Check sheet for the modelled part. Datum: model origin and axes. Units: mm. A direction names the side the tool comes from. Round coordinates to 2 decimals unless told otherwise and drop trailing zeros. Loops run counter-clockwise (first coordinate to the right, second up) from the corner with the lowest first, then second, coordinate; pieces in that order, holes last. Notation, with made-up numbers: (-36, -28.75) - (10, -28.75) arc R27 cw to (10, 8.25) - close; hole circle Ø1 at (-34, 14.25). An arc over 180 degrees is marked (long way). Put each result on its own line as item: value. Start each with the question number.
Item 1: Section check A-A, the plane x = 21. Record the cut outline in (y, z).
Item 2: Section check C-C, the plane z = 23. Record the cut outline in (x, y), and give its area (3 significant figures).
Item 3: Section check D-D, the plane y = 36.5. Record the cut outline in (x, z).
Item 4: Tool access check on faces 4 (the flat face through (21, -19.2, 24)), 5 (the cylindrical face through (37.34, -21.19, 20.89)), 6 (the flat face through (21, -11, 40)). Record the directions out of +Z, -Z, +X, -X, +Y, -Y that give a thin tool (end or side, any length) a straight path to the whole face; none if there is none.
Item 5: Draft check along Y on faces 1 (the cylindrical face through (37.215, 35.125, 1.479)), 2 (the flat face through (16, 19, 3)), 3 (the flat face through (21, -19.2, 45)). Enter one of: pulls with the +Y half, pulls with the -Y half, needs draft (parallel to the pull), parting line crosses it, or undercut.
Item 6: Material ranges on line 1 along X through (y, z) = (-21.25, 23); line 2 along Y through (x, z) = (36.5, 2.1); line 3 along Z through (x, y) = (36, -21), recorded low to high.
Item 7: Section check B-B, the plane y = -16. Record the cut outline in (x, z), and give its area (3 significant figures).
Item 8: Gauge pin test, flat ends, axial feed: pin 1 Ø2 at (x, z) = (28, 22.5) entering from +Y; pin 2 Ø13.5 at (x, y) = (12.5, -6.5) entering from +Z; pin 3 Ø12 at (x, y) = (26, 6.5) entering from +Z. Record the tip position at first contact, or that the pin passes through.
from build123d import *

# Parameters (mm, degrees)
ESQUISSE1_W             = 42
ESQUISSE1_H             = 42
ESQUISSE1_R             = 2.6
ESQUISSE1_R_2           = 1.55
ESQUISSE1_H_2           = 22.2
BOSS_EXTRU_1_DEPTH      = 3
ESQUISSE2_W             = 42
ESQUISSE2_H             = 3
BOSS_EXTRU_2_DEPTH      = 48
BOSS_EXTRU_3_DEPTH      = 42
ENL_V_MAT_EXTRU_4_REACH = 5
ESQUISSE4_R             = 2.5
CHANFREIN1_SIZE         = 1
ESQUISSE5_W             = 42
ESQUISSE5_H             = 10
BOSS_EXTRU_4_DEPTH      = 17


with BuildPart() as part:
    # Esquisse1 → Boss.-Extru.1 (new body)
    with BuildSketch(Plane.XY):
        with Locations((21, 21)):
            Rectangle(ESQUISSE1_W, ESQUISSE1_H)
        with Locations((21, 21)):
            Circle(ESQUISSE1_R, mode=Mode.SUBTRACT)
        with Locations((5.5, 36.5)):
            Circle(ESQUISSE1_R_2, mode=Mode.SUBTRACT)
        with Locations((36.5, 36.5)):
            Circle(ESQUISSE1_R_2, mode=Mode.SUBTRACT)
        with Locations((36.5, 5.5)):
            Circle(ESQUISSE1_R_2, mode=Mode.SUBTRACT)
        with Locations((5.5, 5.5)):
            Circle(ESQUISSE1_R_2, mode=Mode.SUBTRACT)
        with Locations((21, -11.1)):
            Rectangle(ESQUISSE1_W, ESQUISSE1_H_2)
    extrude(amount=BOSS_EXTRU_1_DEPTH)

    # Esquisse2 → Boss.-Extru.2 (add)
    with BuildSketch(Plane.XY.offset(3)):
        with Locations((21, -20.7)):
            Rectangle(ESQUISSE2_W, ESQUISSE2_H)
    extrude(amount=BOSS_EXTRU_2_DEPTH)

    # Esquisse3 → Boss.-Extru.3 (add)
    with BuildSketch(Plane(origin=(42, 0, 0), x_dir=(0, 0, -1), z_dir=(1, 0, 0))):
        Polygon((-3, -4.2), (-18, -19.2), (-3, -19.2), align=None)
    extrude(amount=-BOSS_EXTRU_3_DEPTH)

    # Esquisse4 → Enlèv. mat.-Extru.4 (cut, up to next)
    with BuildSketch(Plane(origin=(0, -19.2, 0), x_dir=(1, 0, 0), z_dir=(0, 1, 0)), mode=Mode.PRIVATE) as enl_v_mat_extru_4_sk1:
        with Locations((5, -23)):
            Circle(ESQUISSE4_R)
    enl_v_mat_extru_4_tool1 = extrude(enl_v_mat_extru_4_sk1.sketch, amount=-ENL_V_MAT_EXTRU_4_REACH, mode=Mode.PRIVATE) & part.part
    add(enl_v_mat_extru_4_tool1.solids().sort_by_distance((5, -19.2, 23))[0], mode=Mode.SUBTRACT)
    # Esquisse4 → Enlèv. mat.-Extru.4 (cut, up to next)
    with BuildSketch(Plane(origin=(0, -19.2, 0), x_dir=(1, 0, 0), z_dir=(0, 1, 0)), mode=Mode.PRIVATE) as enl_v_mat_extru_4_sk2:
        with Locations((36, -23)):
            Circle(ESQUISSE4_R)
    enl_v_mat_extru_4_tool2 = extrude(enl_v_mat_extru_4_sk2.sketch, amount=-ENL_V_MAT_EXTRU_4_REACH, mode=Mode.PRIVATE) & part.part
    add(enl_v_mat_extru_4_tool2.solids().sort_by_distance((36, -19.2, 23))[0], mode=Mode.SUBTRACT)
    # Esquisse4 → Enlèv. mat.-Extru.4 (cut, up to next)
    with BuildSketch(Plane(origin=(0, -19.2, 0), x_dir=(1, 0, 0), z_dir=(0, 1, 0)), mode=Mode.PRIVATE) as enl_v_mat_extru_4_sk3:
        with Locations((36, -46)):
            Circle(ESQUISSE4_R)
    enl_v_mat_extru_4_tool3 = extrude(enl_v_mat_extru_4_sk3.sketch, amount=-ENL_V_MAT_EXTRU_4_REACH, mode=Mode.PRIVATE) & part.part
    add(enl_v_mat_extru_4_tool3.solids().sort_by_distance((36, -19.2, 46))[0], mode=Mode.SUBTRACT)
    # Esquisse4 → Enlèv. mat.-Extru.4 (cut, up to next)
    with BuildSketch(Plane(origin=(0, -19.2, 0), x_dir=(1, 0, 0), z_dir=(0, 1, 0)), mode=Mode.PRIVATE) as enl_v_mat_extru_4_sk4:
        with Locations((5, -46)):
            Circle(ESQUISSE4_R)
    enl_v_mat_extru_4_tool4 = extrude(enl_v_mat_extru_4_sk4.sketch, amount=-ENL_V_MAT_EXTRU_4_REACH, mode=Mode.PRIVATE) & part.part
    add(enl_v_mat_extru_4_tool4.solids().sort_by_distance((5, -19.2, 46))[0], mode=Mode.SUBTRACT)

    # Chanfrein1
    chanfrein1_edges = [part.edges().sort_by_distance(p)[0] for p in [
        (2.5, -19.2, 46),
        (33.5, -19.2, 46),
        (33.5, -19.2, 23),
        (2.5, -19.2, 23),
    ]]
    chamfer(chanfrein1_edges, length=CHANFREIN1_SIZE)

    # Esquisse5 → Boss.-Extru.4 (add)
    with BuildSketch(Plane(origin=(0, -19.2, 0), x_dir=(1, 0, 0), z_dir=(0, 1, 0))):
        with Locations((21, -35)):
            Rectangle(ESQUISSE5_W, ESQUISSE5_H)
    extrude(amount=BOSS_EXTRU_4_DEPTH)


solid = part.part
Check result:
1. outline: (-22.2, 0) - (18.4, 0) - (18.4, 3) - (-4.2, 3) - (-19.2, 18) - (-19.2, 30) - (-2.2, 30) - (-2.2, 40) - (-19.2, 40) - (-19.2, 51) - (-22.2, 51) - close; (23.6, 0) - (42, 0) - (42, 3) - (23.6, 3) - close
2. outline: (0, -22.2) - (2.5, -22.2) - (2.5, -20.2) - (1.5, -19.2) - (0, -19.2) - close; (7.5, -22.2) - (33.5, -22.2) - (33.5, -20.2) - (32.5, -19.2) - (8.5, -19.2) - (7.5, -20.2) - close; (38.5, -22.2) - (42, -22.2) - (42, -19.2) - (39.5, -19.2) - (38.5, -20.2) - close
2. area: 94.0 mm²
3. outline: (0, 0) - (3.95, 0) - (3.95, 3) - (0, 3) - close; (7.05, 0) - (34.95, 0) - (34.95, 3) - (7.05, 3) - close; (38.05, 0) - (42, 0) - (42, 3) - (38.05, 3) - close
4. face 4: +X, -X, +Y
4. face 5: +Y, -Y
4. face 6: +Z, +X, -X, +Y
5. face 1: undercut
5. face 2: needs draft
5. face 3: pulls with the +Y half
6. line 1: 0 to 2.5, 7.5 to 33.5, 38.5 to 42
6. line 2: -22.2 to 3.95, 7.05 to 34.95, 38.05 to 42
6. line 3: 0 to 20.5, 25.5 to 43.5, 48.5 to 51
7. outline: (0, 0) - (42, 0) - (42, 14.8) - (0, 14.8) - close; (0, 30) - (42, 30) - (42, 40) - (0, 40) - close
7. area: 1,040 mm²
8. pin 1: y = -19.2
8. pin 2: z = 40
8. pin 3: z = 3
